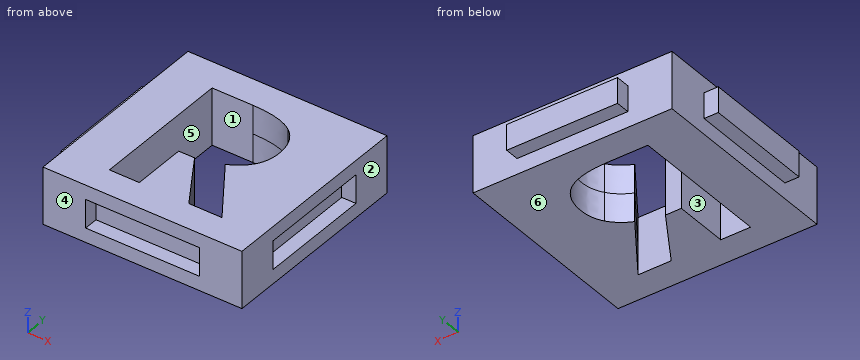
```python
from build123d import *

# Parameters (mm, degrees)
F0_W     = 35.56
F0_H     = 35.56
F1_DEPTH = 5.08
F2_W     = 19.812
F2_H     = 4.572
F3_DEPTH = 2.54
F4_W     = 19.812
F4_H     = 4.572
F5_DEPTH = 2.54
F6_W     = 20.32
F6_H     = 5.08
F7_DEPTH = 2.54
F8_W     = 20.32
F8_H     = 5.08
F9_DEPTH = 2.54


with BuildPart() as f1:
    # F0 (on Top) → F1 (new body, symmetric)
    with BuildSketch(Plane.XY):
        Rectangle(F0_W, F0_H)
        with BuildLine():
            Line((-1.438671875, -3.0371961806), (-4.2774305556, -3.0371961806))
            Line((-4.2774305556, -3.0371961806), (-4.2774305556, -12.7))
            Line((-4.2774305556, -12.7), (-9.6187065972, -12.7))
            Line((-9.6187065972, -12.7), (-9.6187065972, 12.4850260417))
            Line((-9.6187065972, 12.4850260417), (-2.28203125, 12.4850260417))
            add(Edge.make_bspline(
                [(-2.28203125, 12.4850260417), (2.8552951389, 12.4850260417), (5.3164713542, 10.61640625)],
                knots=[0, 0, 0, 1, 1, 1], degree=2))
            add(Edge.make_bspline(
                [(5.3164713542, 10.61640625), (7.7776475694, 8.7477864583), (7.7776475694, 4.9388888889)],
                knots=[0, 0, 0, 1, 1, 1], degree=2))
            add(Edge.make_bspline(
                [(7.7776475694, 4.9388888889), (7.7776475694, 2.7174913194), (6.5567057292, 0.9866753472)],
                knots=[0, 0, 0, 1, 1, 1], degree=2))
            add(Edge.make_bspline(
                [(6.5567057292, 0.9866753472), (5.3357638889, -0.744140625), (3.0923177083, -1.7253038194)],
                knots=[0, 0, 0, 1, 1, 1], degree=2))
            add(Edge.make_bspline(
                [(3.0923177083, -1.7253038194), (8.780859375, -10.21953125), (10.5006510417, -12.7)],
                knots=[0, 0, 0, 1, 1, 1], degree=2))
            Line((10.5006510417, -12.7), (4.5750868056, -12.7))
            Line((4.5750868056, -12.7), (-1.438671875, -3.0371961806))
        make_face(mode=Mode.SUBTRACT)
    extrude(amount=F1_DEPTH, both=True)

    # F2 (on face) → F3 (join)
    with BuildSketch(Plane(origin=(0, 17.78, 0), x_dir=(-1, 0, 0), z_dir=(0, 1, 0))):
        Rectangle(F2_W, F2_H)
    extrude(amount=F3_DEPTH)

    # F4 (on face) → F5 (join)
    with BuildSketch(Plane(origin=(-17.78, 0, 0), x_dir=(0, -1, 0), z_dir=(-1, 0, 0))):
        Rectangle(F4_W, F4_H)
    extrude(amount=F5_DEPTH)

    # F6 (on face) → F7 (cut)
    with BuildSketch(Plane.XZ.offset(17.78)):
        Rectangle(F6_W, F6_H)
    extrude(amount=-F7_DEPTH, mode=Mode.SUBTRACT)

    # F8 (on face) → F9 (cut)
    with BuildSketch(Plane.YZ.offset(17.78)):
        Rectangle(F8_W, F8_H)
    extrude(amount=-F9_DEPTH, mode=Mode.SUBTRACT)


solid = f1.part
```
Part model, mm, in its own coordinate system. Face numbers are marked on the shaded views. A direction names the side the tool comes from. Round coordinates to 2 decimals unless told otherwise and drop trailing zeros. Write each loop counter-clockwise with the first axis right and the second up, starting at its lowest first coordinate (ties: lowest second). Pieces come first, ordered by that corner, then holes. Notation, with made-up numbers: (36.25, 16) -> (78.25, 16) arc R22 ccw to (78.25, 51) -> close; hole circle Ø8 at (-22, 64.5). An arc over 180 degrees is marked (long way). Return JSON: item names as keys, results as strings. Group by question number.
Q1. Saw through at B-B on y = -14. Write the cut outline in (x, z), plus the area to 3 significant figures.
Q2. Mould opens along Y. For the marked faces 3, 4, 5 and 6 say: pulls with the +Y half, pulls with the -Y half, needs draft (parallel to the pull), parting line crosses it, or undercut.
Q3. Probe L1, parallel to Y at x = 6, z = 1; L2, parallel to X at y = -12, z = -1.75; L3, parallel to Y at x = -6, z = 1. List the from-to ranges inside material, lowest first. Write a range as [from, to].
Q4. Pin check, flat tips, straight feed: pin 1 (0.8 mm diameter, centred on x = 1.5, y = 19.5, fed in from -Z); pin 2 (1 mm diameter, centred on y = 9.5, z = 3.5, fed in from -X); pin 3 (3 mm diameter, centred on x = -19.5, y = 1.5, fed in from +Z). Stop position of each tip, or through.
Q5. Saw through at A-A on x = -7. Write the cut outline in (y, z), plus the area to 3 significant figures.
Q6. Saw through at D-D on y = -7.5. State how many separate pieces and enclosed holes the cut face has, plus the area to 3 significant figures.
Q7. Which spindle directions (+Z, -Z, +X, -X, +Y, -Y) get a long thin tool onto all of the face, cutting with end or side? Do the marked faces 1 and 2. Say none if no direction does.
Answer:
{
 "1": {"outline": "(-17.78, -5.08) -> (17.78, -5.08) -> (17.78, 5.08) -> (-17.78, 5.08) -> close", "area": "361 mm2"},
 "2": {"face 3": "undercut", "face 4": "pulls with the -Y half", "face 5": "undercut", "face 6": "needs draft"},
 "3": {"L1": "[-15.24, -12.7], [-6.06, 0.29], [10.01, 20.32]", "L2": "[-17.78, -9.62], [-4.28, 4.14], [10.02, 17.78]", "L3": "[-15.24, -12.7], [12.49, 20.32]"},
 "4": {"pin 1": "z = -2.29", "pin 2": "x = -17.78", "pin 3": "z = 2.29"},
 "5": {"outline": "(-17.78, -5.08) -> (-12.7, -5.08) -> (-12.7, 5.08) -> (-17.78, 5.08) -> (-17.78, 2.54) -> (-15.24, 2.54) -> (-15.24, -2.54) -> (-17.78, -2.54) -> close; (12.49, -5.08) -> (17.78, -5.08) -> (17.78, -2.29) -> (20.32, -2.29) -> (20.32, 2.29) -> (17.78, 2.29) -> (17.78, 5.08) -> (12.49, 5.08) -> close", "area": "104 mm2"},
 "6": {"separate pieces": "3", "enclosed holes": "0", "area": "249 mm2"},
 "7": {"face 1": "+Z, -Z", "face 2": "+Z, -Z, +X, +Y, -Y"}
}
